Model file for the job. Use its own axes, mm. Coordinates: 2 decimals unless noted, no trailing zeros. Write each loop counter-clockwise with the first axis right and the second up, starting at its lowest first coordinate (ties: lowest second). Pieces come first, ordered by that corner, then holes. Notation, with made-up numbers: (-27, 23) -> (14, 23) arc R5 cw to (14, 31) -> close; hole circle Ø3 at (55, -12.5). An arc over 180 degrees is marked (long way). Answer as a JSON object with one key per item and string values. Group by question number.
from build123d import *

# Parameters (mm, degrees)
SKETCH1_W                 = 74.549
SKETCH1_H                 = 74.549
SKETCH1_R                 = 26.67
BOSS_EXTRUDE1_DEPTH       = 0.762
BOSS_EXTRUDE1_DEPTH_BACK  = 1.778
SKETCH2_R                 = 3.302
CUT_EXTRUDE1_DEPTH        = 3.54
MIRROR2_COPY_1_SKETCH_R   = 3.302
MIRROR2_COPY_1_DEPTH      = 3.54
SKETCH14_OUTSIDE_W        = 97.642
SKETCH14_OUTSIDE_H        = 97.642
SKETCH14_OUTSIDE_R        = 33.2486
CUT_EXTRUDE6_DEPTH        = 3.54
SKETCH15_W                = 6.35
SKETCH15_H                = 8.89
CUT_EXTRUDE7_DEPTH        = 1.524
FILLET2_R                 = 1.27
CIRPATTERN2_COUNT         = 7
FILLET2_OF_CIRPATTERN2_R  = 1.27
SKETCH16_R                = 0.0127
CUT_EXTRUDE8_DEPTH        = 3.54
F_0_80_TAPPED_HOLE3_D     = 1.19126
F_0_80_TAPPED_HOLE3_DEPTH = 4.064
F_0_80_TAPPED_HOLE3_TIP   = 0.357890611


with BuildPart() as part:
    # Sketch1 → Boss-Extrude1 (new body, two sides)
    with BuildSketch(Plane.XY) as boss_extrude1_sk:
        Rectangle(SKETCH1_W, SKETCH1_H)
        Circle(SKETCH1_R, mode=Mode.SUBTRACT)
    extrude(amount=BOSS_EXTRUDE1_DEPTH)
    extrude(boss_extrude1_sk.sketch, amount=-BOSS_EXTRUDE1_DEPTH_BACK)

    # Sketch2 → Cut-Extrude1 (cut, through all)
    with BuildSketch(Plane.XY.offset(0.762)):
        with Locations((-31.75, 31.75)):
            Circle(SKETCH2_R)
    cut_extrude1 = extrude(amount=-CUT_EXTRUDE1_DEPTH, mode=Mode.SUBTRACT)

    # Mirror1: Cut-Extrude1 across plane
    add(cut_extrude1.mirror(Plane(origin=(0, 0, 0), x_dir=(0, 0, 1), z_dir=(1, 0, 0))), mode=Mode.SUBTRACT)

    # Mirror2: Cut-Extrude1 across plane
    add(cut_extrude1.mirror(Plane.ZX), mode=Mode.SUBTRACT)

    # Mirror2 copy 1 sketch → Mirror2 copy 1 (cut, through all)
    with BuildSketch(Plane(origin=(0, 0, 0.762), x_dir=(-1, 0, 0), z_dir=(0, 0, 1))):
        with Locations((-31.75, 31.75)):
            Circle(MIRROR2_COPY_1_SKETCH_R)
    extrude(amount=-MIRROR2_COPY_1_DEPTH, mode=Mode.SUBTRACT)

    # Sketch14 outside → Cut-Extrude6 (cut, through all)
    with BuildSketch(Plane.XY.offset(0.762)):
        Rectangle(SKETCH14_OUTSIDE_W, SKETCH14_OUTSIDE_H)
        Circle(SKETCH14_OUTSIDE_R, mode=Mode.SUBTRACT)
    extrude(amount=-CUT_EXTRUDE6_DEPTH, mode=Mode.SUBTRACT)

    # Sketch15 → Cut-Extrude7 (cut)
    with BuildSketch(Plane.XY.offset(0.762)):
        with Locations((0, 25.7175)):
            Rectangle(SKETCH15_W, SKETCH15_H)
    cut_extrude7 = extrude(amount=-CUT_EXTRUDE7_DEPTH, mode=Mode.SUBTRACT)

    # Fillet2
    fillet2_edges = [part.edges().sort_by_distance(p)[0] for p in [
        (3.175, 30.1625, 0),
        (-3.175, 30.1625, 0),
    ]]
    fillet(fillet2_edges, radius=FILLET2_R)

    # CirPattern2: Cut-Extrude7 ×7 about axis
    cirpattern2_axis = Axis((0, 0, 0), (0, 0, 1))
    for i in range(1, CIRPATTERN2_COUNT):
        add(cut_extrude7.rotate(cirpattern2_axis, i * 360 / CIRPATTERN2_COUNT), mode=Mode.SUBTRACT)

    # Fillet2 of CirPattern2
    fillet2_of_cirpattern2_edges = [part.edges().sort_by_distance(p)[0] for p in [
        (-21.602411969, 21.288326105, 0),
        (-25.561572211, 16.323696192, 0),
        (-30.112767116, -3.616391549, 0),
        (-28.699759186, -9.807183792, 0),
        (-15.947594437, -25.797892606, 0),
        (-10.226442126, -28.55305435, 0),
        (10.226442126, -28.55305435, 0),
        (15.947594437, -25.797892606, 0),
        (28.699759186, -9.807183792, 0),
        (30.112767116, -3.616391549, 0),
        (25.561572211, 16.323696192, 0),
        (21.602411969, 21.288326105, 0),
    ]]
    fillet(fillet2_of_cirpattern2_edges, radius=FILLET2_OF_CIRPATTERN2_R)

    # Sketch16 → Cut-Extrude8 (cut, through all)
    with BuildSketch(Plane.XY.offset(0.762)):
        with Locations((-15.24, 26.396454307)):
            Circle(SKETCH16_R)
    cut_extrude8 = extrude(amount=-CUT_EXTRUDE8_DEPTH, mode=Mode.SUBTRACT)

    # Mirror4: Cut-Extrude8 across plane
    add(cut_extrude8.mirror(Plane(origin=(0, 0, 0), x_dir=(0, 0, 1), z_dir=(1, 0, 0))), mode=Mode.SUBTRACT)

    # 0-80 Tapped Hole3
    with Locations(Plane.XY.offset(0.762)):
        with Locations((-15.24, 26.396454307), (15.24, 26.396454307)):
            Hole(F_0_80_TAPPED_HOLE3_D / 2, depth=F_0_80_TAPPED_HOLE3_DEPTH)
            with Locations((0, 0, -(F_0_80_TAPPED_HOLE3_DEPTH + F_0_80_TAPPED_HOLE3_TIP / 2))):  # 118° drill point
                Cone(0, F_0_80_TAPPED_HOLE3_D / 2, F_0_80_TAPPED_HOLE3_TIP, mode=Mode.SUBTRACT)


solid = part.part
(1) Pull direction X, two halves, no side cores. Call faces 1 (the face through (23.565, 18.827, 0.011)), 2 (the face through (-19.65, 19.73, 0.01)): released by +X, released by -X, zero draft, split by the parting line, or undercut.
(2) Cut at A-A on x = 0. List the corners of the cut face in (y, z), plus the area to 3 significant figures.
(3) Pin check, flat tips, straight feed: pin 1 (0.8 mm diameter, centred on y = 27.5, z = -0.5, fed in from +X); pin 2 (1 mm diameter, centred on x = 9, z = 0, fed in from +Y); pin 3 (1.2 mm diameter, centred on y = 28, z = 0, fed in from -X). Stop position of each tip, or through.
(4) Cut at B-B on y = -15. List the corners of the cut face in (x, z), plus the area to 3 significant figures.
(5) Cut at C-C on y = 16.5. List the corners of the cut face in (x, z).
(6) Wall check: probe 1 along Y at (x, z) = (0, -0.7); probe 2 along Y at (x, z) = (15.24, -0.6); probe 3 along X at (y, z) = (4, -0.5). Give the ranges that are in metal, low to high.
(7) Cut at D-D on x = 17.5. List the corners of the cut face in (y, z), plus the area to 3 significant figures.
Results found:
{
 "1": {"face 1": "undercut", "face 2": "undercut"},
 "2": {"outline": "(-33.25, -1.78) -> (-26.67, -1.78) -> (-26.67, 0.76) -> (-33.25, 0.76) -> close; (26.67, -1.78) -> (33.25, -1.78) -> (33.25, 0.76) -> (30.16, 0.76) -> (30.16, -0.76) -> (26.67, -0.76) -> close", "area": "28.1 mm²"},
 "3": {"pin 1": "stops at x = 19.26", "pin 2": "stops at y = 32.14", "pin 3": "stops at x = -18.83"},
 "4": {"outline": "(-29.67, -1.78) -> (-22.05, -1.78) -> (-22.05, 0.76) -> (-29.67, 0.76) -> close; (22.05, -1.78) -> (29.67, -1.78) -> (29.67, 0.76) -> (22.05, 0.76) -> close", "area": "38.7 mm²"},
 "5": {"outline": "(-28.87, -1.78) -> (-20.95, -1.78) -> (-20.95, -0.76) -> (-25.05, -0.76) -> (-25.05, 0.76) -> (-28.87, 0.76) -> close; (20.95, -1.78) -> (28.87, -1.78) -> (28.87, 0.76) -> (25.05, 0.76) -> (25.05, -0.76) -> (20.95, -0.76) -> close"},
 "6": {"probe 1": "y = -33.25 to -26.67, 30.16 to 33.25", "probe 2": "y = -29.55 to -26, -24.33 to -21.89, 21.89 to 25.8, 26.99 to 29.55", "probe 3": "x = -33.01 to -26.37, 26.37 to 33.01"},
 "7": {"outline": "(-28.27, -1.78) -> (-20.13, -1.78) -> (-20.13, 0.76) -> (-28.27, 0.76) -> close; (20.13, -1.78) -> (28.27, -1.78) -> (28.27, 0.76) -> (20.13, 0.76) -> close", "area": "41.4 mm²"}
}
